For this review, take the finished solid that the model builds, in its own axes (mm). Face numbers are marked on the shaded views. A direction names the side the tool comes from. Round coordinates to 2 decimals unless told otherwise and drop trailing zeros. Write each loop counter-clockwise with the first axis right and the second up, starting at its lowest first coordinate (ties: lowest second). Pieces come first, ordered by that corner, then holes. Notation, with made-up numbers: (11, 49) - (37, 49) arc R9 ccw to (37, 56) - close; hole circle Ø6 at (37.5, 8). An arc over 180 degrees is marked (long way). One line per item, written item: value. Start each with the question number.
Q1. Tool access review of the marked faces 4 and 5: name each direction out of +Z, -Z, +X, -X, +Y, -Y from which nothing blocks a thin tool from reaching the whole face with its end or side.
Q2. Add section D-D on x = 8. Write out the cut boundary in (y, z).
Q3. Add section C-C on z = -3. Write out the cut boundary in (x, y), and give its area (3 significant figures).
Q4. Mouldability with a two-part tool opening along Y and no side actions: class the marked faces 1, 2 and 3 as +Y half, -Y half, draft (parallel to the pull), parting line (faces both ways), or undercut.
Q5. Clearance check with flat-ended pins moving along their axes: pin 1 Ø2 at (y, z) = (13.5, -3.5) entering from -X; pin 2 Ø3 at (x, z) = (-5, -12) entering from -Y; pin 3 Ø6 at (x, z) = (9, -4) entering from +Y. State where each tip first meets the part, or that it passes through.
Q6. Add section A-A on y = 0. Write out the cut boundary in (x, z), and give its area (4 significant figures).
Q7. For probe 1 along Y at (x, z) = (0, -7.25); probe 2 along Y at (x, z) = (0, -13); probe 3 along Z at (x, y) = (-19.5, 23), list the stretches that pass through material, from the lowest coordinate up.
```python
from build123d import *

# Parameters (mm, degrees)
SKETCH_3_R          = 15
EXTRUDE_1_DEPTH     = 7
SKETCH_4_R          = 3.25
CUT_EXTRUDE_1_DEPTH = 18


with BuildPart() as part:
    # Эскиз2 → Повернуть1 (revolve)
    with BuildSketch(Plane(origin=(0, 0, 0), x_dir=(0, 0, -1), z_dir=(1, 0, 0))):
        Polygon((0, 0), (0, 30.5), (1.5, 30.5), (1.5, 28.5), (8.5, 28.5), (8.5, 30.5), (10, 30.5), (10, 0), align=None)
    revolve(axis=Axis((0, 0, -10), (0, 0, 1)))

    # Эскиз3 → Бобышка-Вытянуть1 (add)
    with BuildSketch(Plane(origin=(0, 0, -10), x_dir=(-1, 0, 0), z_dir=(0, 0, -1))):
        Circle(SKETCH_3_R)
    extrude(amount=EXTRUDE_1_DEPTH)

    # Эскиз4 → Вырез-Вытянуть1 (cut, through all)
    with BuildSketch(Plane(origin=(0, 0, -17), x_dir=(-1, 0, 0), z_dir=(0, 0, -1))):
        Circle(SKETCH_4_R)
    extrude(amount=-CUT_EXTRUDE_1_DEPTH, mode=Mode.SUBTRACT)


solid = part.part
```
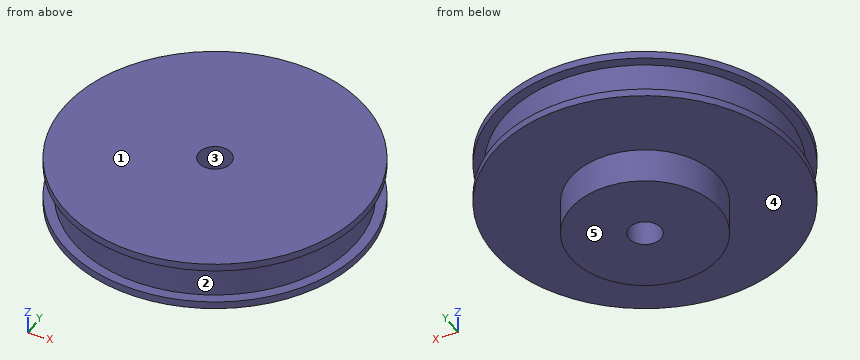
Result set:
1. face 4: -Z
1. face 5: -Z, +X, -X, +Y, -Y
2. outline: (-29.43, -10) - (-12.69, -10) - (-12.69, -17) - (12.69, -17) - (12.69, -10) - (29.43, -10) - (29.43, -8.5) - (27.35, -8.5) - (27.35, -1.5) - (29.43, -1.5) - (29.43, 0) - (-29.43, 0) - (-29.43, -1.5) - (-27.35, -1.5) - (-27.35, -8.5) - (-29.43, -8.5) - close
3. outline: circle Ø57 at (0, 0); hole circle Ø6.5 at (0, 0)
3. area: 2,520 mm^2
4. face 1: draft
4. face 2: parting line
4. face 3: undercut
5. pin 1: stops at x = -25.61
5. pin 2: stops at y = -14.59
5. pin 3: stops at y = 29.6
6. outline: (-30.5, -10) - (-15, -10) - (-15, -17) - (-3.25, -17) - (-3.25, 0) - (-30.5, 0) - (-30.5, -1.5) - (-28.5, -1.5) - (-28.5, -8.5) - (-30.5, -8.5) - close; (3.25, -17) - (15, -17) - (15, -10) - (30.5, -10) - (30.5, -8.5) - (28.5, -8.5) - (28.5, -1.5) - (30.5, -1.5) - (30.5, 0) - (3.25, 0) - close
6. area: 681.5 mm^2
7. probe 1: y = -28.5 to -3.25, 3.25 to 28.5
7. probe 2: y = -15 to -3.25, 3.25 to 15
7. probe 3: z = -10 to -8.5, -1.5 to 0
